Model file for the job. Use its own axes, mm. A direction names the side the tool comes from. Coordinates: 2 decimals unless noted, no trailing zeros. Order: outer loops, then holes, each group sorted by start corner. A loop starts at its lowest first (then second) coordinate and runs counter-clockwise, first axis right, second up. Notation, with made-up numbers: M 10.5,78.25 L 59.5,78.25 A32 ccw 59.5,112.25 Z; hole C 31.25,-7 d5. An arc over 180 degrees is marked long. Return JSON: item names as keys, results as strings.
```python
from build123d import *

# Parameters (mm, degrees)
SKETCH1_R           = 9.525
BOSS_EXTRUDE1_DEPTH = 6.35
SKETCH2_R           = 4.7625
BOSS_EXTRUDE2_DEPTH = 19.05
SKETCH3_R           = 6.35
BOSS_EXTRUDE3_DEPTH = 19.05


with BuildPart() as part:
    # Sketch1 → Boss-Extrude1 (new, symmetric)
    with BuildSketch(Plane(origin=(0, 0, 0), x_dir=(0, 0, -1), z_dir=(1, 0, 0))):
        Circle(SKETCH1_R)
    extrude(amount=BOSS_EXTRUDE1_DEPTH, both=True)

    # Sketch2 → Boss-Extrude2 (add)
    with BuildSketch(Plane(origin=(6.35, 0, 0), x_dir=(0, 0, -1), z_dir=(1, 0, 0))):
        with Locations(Location((0, 0, 0), (0, 0, 180))):
            Circle(SKETCH2_R)
    extrude(amount=BOSS_EXTRUDE2_DEPTH)

    # Sketch3 → Boss-Extrude3 (add)
    with BuildSketch(Plane.ZY.offset(6.35)):
        with Locations(Location((0, 0, 0), (0, 0, 180))):
            Circle(SKETCH3_R)
    extrude(amount=BOSS_EXTRUDE3_DEPTH)


solid = part.part
```
Item 1: Wall check: line 1 (X direction, y = -6, z = 5.75); line 2 (Y direction, x = 15.5, z = -0.25); line 3 (X direction, y = -4.25, z = 4.5). Give the ranges that are in metal, low to high.
Check result:
{"line 1": "x = -6.35 to 6.35", "line 2": "y = -4.76 to 4.76", "line 3": "x = -25.4 to 6.35"}
Item 2: 3-axis set-ups, long thin cutter, end or side, ignore diameter. For faces 1 (the flat face through (-25.4, 0, 0)), 2 (the cylindrical face through (-15.742, 5.634, -2.93)), 3 (the flat face through (6.35, 2.3, 4.4)): which of +Z, -Z, +X, -X, +Y, -Y reach the whole face in a straight line?
Check result:
{"face 1": "+Z, -Z, -X, +Y, -Y", "face 2": "-X", "face 3": "+X"}
Item 3: Saw through at D-D (z = -5.25). Write the cut outline in (x, y).
Check result:
{"outline": "M -25.4,-3.57 L -6.35,-3.57 L -6.35,-7.95 L 6.35,-7.95 L 6.35,7.95 L -6.35,7.95 L -6.35,3.57 L -25.4,3.57 Z"}
Item 4: Drop flat-ended pins along their axis: pin 1 Ø4 at (x, z) = (19.5, 4.5) entering from -Y; pin 2 Ø3 at (x, z) = (-3.5, 1) entering from +Y (3 decimals); pin 3 Ø10 at (x, z) = (16.5, -4.5) entering from -Y; pin 4 Ø6 at (x, y) = (-19.5, 0) entering from +Z. Give the stop position or say it passes through.
Check result:
{"pin 1": "stops at y = -4.05", "pin 2": "stops at y = 9.525", "pin 3": "stops at y = -4.76", "pin 4": "stops at z = 6.35"}
Item 5: Saw through at C-C (x = -7.5). Write the cut outline in (y, z), and give its area (3 significant figures).
Check result:
{"outline": "C 0,0 d12.7", "area": "127 mm2"}
